from build123d import *

# Parameters (mm, degrees)
SUPERFICIE_EXTRUIR1_1_DEPTH = 40
DAR_ESPESOR1_T1             = 3
EXTRUIR1_DEPTH              = 20
EXTRUIR1_DEPTH_BACK         = 23
CROQUIS2_R                  = 5
CROQUIS3_R                  = 5
EXTRUIR2_DEPTH              = 20


with BuildPart() as body_1:
    # Superficie-Extruir1: a surface, the sketch's curves swept straight by 40 mm
    with BuildLine(Plane.XY, mode=Mode.PRIVATE) as superficie_extruir1_1_path:
        Line((0, -70), (0, 0))
        Line((0, 0), (-40, 0))
    superficie_extruir1_1 = Shell.extrude(superficie_extruir1_1_path.wire(), (0 * SUPERFICIE_EXTRUIR1_1_DEPTH, 0 * SUPERFICIE_EXTRUIR1_1_DEPTH, 1 * SUPERFICIE_EXTRUIR1_1_DEPTH))
    add(Solid.thicken(superficie_extruir1_1, DAR_ESPESOR1_T1))

    # Croquis2 → Extruir1 (add, two sides: drawn at the far end of the back side and taken through both)
    with BuildSketch(Plane(origin=(0, 0, 0), x_dir=(1, 0, 0), z_dir=(0, 1, 0)).offset(-EXTRUIR1_DEPTH_BACK)):
        with Locations(Location((-20, -20, 0), (0, 0, 180))):
            Circle(CROQUIS2_R)
    extrude(amount=EXTRUIR1_DEPTH + EXTRUIR1_DEPTH_BACK)

    # Croquis3 → Extruir2 (cut)
    with BuildSketch(Plane.ZY.offset(3)):
        with Locations(Location((20, -56.5, 0), (0, 0, 270))):
            Circle(CROQUIS3_R)
        with Locations(Location((20, -16.5, 0), (0, 0, 90))):
            Circle(CROQUIS3_R)
    extrude(amount=-EXTRUIR2_DEPTH, mode=Mode.SUBTRACT)


solid = body_1.part
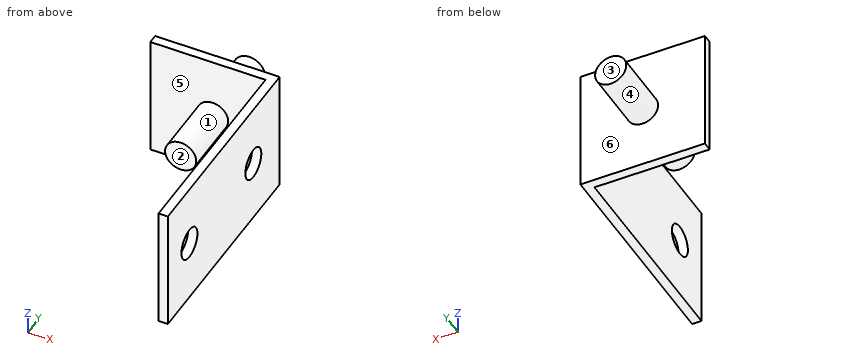
Check sheet for the modelled part. Datum: model origin and axes. Units: mm. Face numbers are marked on the shaded views. A direction names the side the tool comes from. Coordinates: 2 decimals unless noted, no trailing zeros. Write each loop counter-clockwise with the first axis right and the second up, starting at its lowest first coordinate (ties: lowest second). Pieces come first, ordered by that corner, then holes.
Item 1: Cross-section at D-D on y = -16.5. Record the boundary of the cut face in (x, z).
Numbers:
outline: circle Ø10 at (-20, 20); (-3, 0) - (0, 0) - (0, 15) - (-3, 15) - close; (-3, 25) - (0, 25) - (0, 40) - (-3, 40) - close
Item 2: Cross-section at A-A on y = -56.5. Record the boundary of the cut face in (x, z).
Numbers:
outline: (-3, 0) - (0, 0) - (0, 15) - (-3, 15) - close; (-3, 25) - (0, 25) - (0, 40) - (-3, 40) - close
Item 3: Mould release check, pull along X, two halves, no side actions. Record for the marked faces 4, 5 and 6: released by +X, released by -X, zero draft, split by the parting line, or undercut.
Numbers:
face 4: split by the parting line
face 5: undercut
face 6: zero draft
Item 4: Cross-section at C-C on x = -20. Record the boundary of the cut face in (y, z), then the cut area to 3 significant figures.
Numbers:
outline: (-23, 15) - (-3, 15) - (-3, 0) - (0, 0) - (0, 15) - (20, 15) - (20, 25) - (0, 25) - (0, 40) - (-3, 40) - (-3, 25) - (-23, 25) - close
area: 520 mm2
Item 5: Scan lines: probe 1 along Z at (x, y) = (-1.65, -56.5); probe 2 along X at (y, z) = (-53, 11). Record each from-to range of solid material in increasing order.
Numbers:
probe 1: z = 0 to 15, 25 to 40
probe 2: x = -3 to 0
Item 6: Cross-section at B-B on z = 20. Record the boundary of the cut face in (x, y), then the cut area to 3 significant figures.
Numbers:
outline: (-40, -3) - (-25, -3) - (-25, -23) - (-15, -23) - (-15, -3) - (-3, -3) - (-3, -11.5) - (0, -11.5) - (0, 0) - (-15, 0) - (-15, 20) - (-25, 20) - (-25, 0) - (-40, 0) - close; (-3, -70) - (0, -70) - (0, -61.5) - (-3, -61.5) - close; (-3, -51.5) - (0, -51.5) - (0, -21.5) - (-3, -21.5) - close
area: 661 mm2
Item 7: Access from +Z, -Z, +X, -X, +Y, -Y to the whole of each face (thin tool, end or side, straight path). Record for the marked faces 1, 2 and 3.
Numbers:
face 1: -Y
face 2: +Z, -Z, -X, -Y
face 3: +Z, -Z, +X, -X, +Y
Item 8: Depth check by flat-ended pin: pin 1 Ø1.5 at (x, y) = (-17.5, -19.5) entering from +Z; pin 2 Ø8 at (x, z) = (-18.5, 22) entering from -Y; pin 3 Ø4 at (x, z) = (-12.5, 33.5) entering from +Y. Enter the tip coordinate at first touch or a pass-through.
Numbers:
pin 1: stops at z = 24.68
pin 2: stops at y = -23
pin 3: stops at y = 0
